The drawing under review shows one solid part. Ordinate dimensions are in mm from its lowest x, y, z. Give positions to 0.01 mm unless a question says otherwise; leave off trailing zeros. Write each loop counter-clockwise with the first axis right and the second up, starting at its lowest first coordinate (ties: lowest second). Pieces come first, ordered by that corner, then holes. Notation, with made-up numbers: (31.5, 75.25) -> (62.5, 75.25) arc R13 ccw to (62.5, 84.25) -> close; hole circle Ø2 at (25, -27). An arc over 180 degrees is marked (long way). Use CSV: the item, a comma, the result in double quotes.
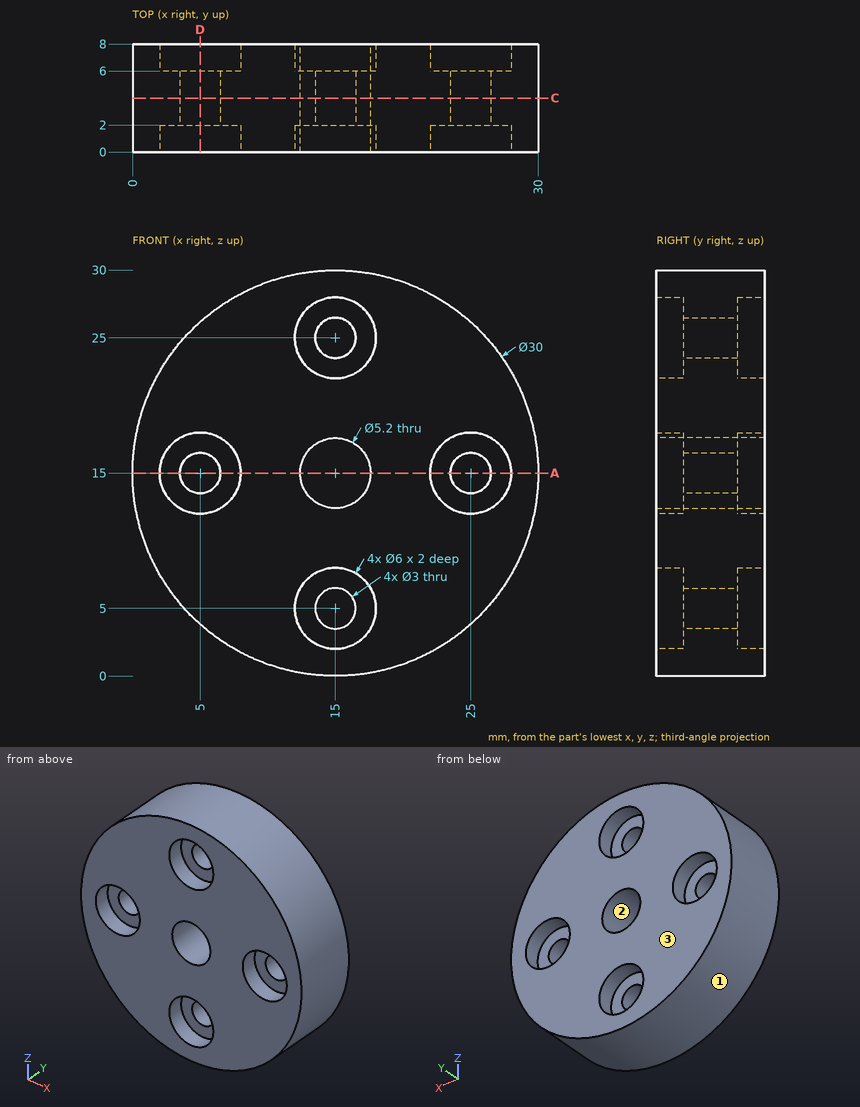
(1) Mouldability with a two-part tool opening along X and no side actions: class the marked faces 1, 2 and 3 as +X half, -X half, draft (parallel to the pull), parting line (faces both ways), or undercut.
Established:
face 1,"parting line"
face 2,"undercut"
face 3,"draft"
(2) Take a section at C-C (y = 4). Write out the cut boundary in (x, z), then the cut area to 3 significant figures.
Established:
outline,"circle Ø30 at (15, 15); hole circle Ø3 at (5, 15); hole circle Ø5.2 at (15, 15); hole circle Ø3 at (15, 5); hole circle Ø3 at (15, 25); hole circle Ø3 at (25, 15)"
area,"657 mm2"
(3) For line 1 along X through (y, z) = (5.2, 15); line 2 along X through (y, z) = (0.6, 15); line 3 along Z through (x, y) = (16, 7), list the stretches that pass through material, from the lowest coordinate up. Write a range as [from, to].
Established:
line 1,"x = [0, 3.5], [6.5, 12.4], [17.6, 23.5], [26.5, 30]"
line 2,"x = [0, 2], [8, 12.4], [17.6, 22], [28, 30]"
line 3,"z = [0.03, 2.17], [7.83, 12.6], [17.4, 22.17], [27.83, 29.97]"
(4) Take a section at A-A (z = 15). State how many separate pieces and enclosed holes the cut face has, then the cut area to 3 significant figures.
Established:
separate pieces,"4"
enclosed holes,"0"
area,"126 mm2"
(5) Take a section at D-D (x = 5). Write out the cut boundary in (y, z).
Established:
outline,"(0, 3.82) -> (8, 3.82) -> (8, 12) -> (6, 12) -> (6, 13.5) -> (2, 13.5) -> (2, 12) -> (0, 12) -> close; (0, 18) -> (2, 18) -> (2, 16.5) -> (6, 16.5) -> (6, 18) -> (8, 18) -> (8, 26.18) -> (0, 26.18) -> close"
(6) Clearance check with flat-ended pins moving along their axes: pin 1 (3.5 mm diameter, centred on x = 5, z = 15, fed in from -Y); pin 2 (1.8 mm diameter, centred on x = 15, z = 25, fed in from -Y); pin 3 (4 mm diameter, centred on y = 4.5, z = 8, fed in from +X); pin 4 (4 mm diameter, centred on y = 2.5, z = 25, fed in from -X). State where each tip first meets the part, or that it passes through.
Established:
pin 1,"stops at y = 2"
pin 2,"passes through"
pin 3,"stops at x = 29.14"
pin 4,"stops at x = 2.31"
